Part model, mm, in its own coordinate system. Give positions to 0.01 mm unless a question says otherwise; leave off trailing zeros. Order: outer loops, then holes, each group sorted by start corner. A loop starts at its lowest first (then second) coordinate and runs counter-clockwise, first axis right, second up. Notation, with made-up numbers: M -8,39 L -4,39 A8 ccw -4,53 Z; hole C 18.25,31.5 d11. An arc over 180 degrees is marked long. Answer as a JSON object with one key per item and string values.
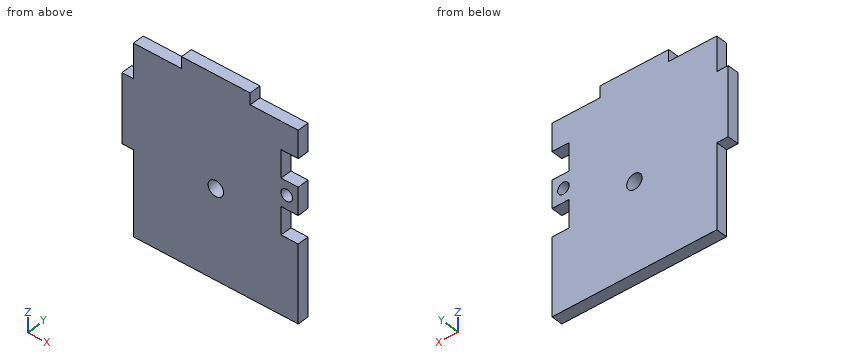
from build123d import *

# Parameters (mm, degrees)
BOSS_EXTRUDE1_DEPTH  = 3.175
M3_CLEARANCE_HOLE1_D = 3.2
SKETCH4_R            = 2.1336
CUT_EXTRUDE1_DEPTH   = 70.232936135


with BuildPart() as part:
    # Sketch1 → Boss-Extrude1 (new body)
    with BuildSketch(Plane(origin=(0, 0, 0), x_dir=(1, 0, 0), z_dir=(0, 1, 0))):
        Polygon((0, 0), (13.335, 0), (13.335, -3.175), (32.385, -3.175), (32.385, 0), (45.72, 0), (45.72, 7.62), (40.9575, 7.62), (40.9575, 15.24), (45.72, 15.24), (45.72, 22.86), (40.9575, 22.86), (40.9575, 30.48), (45.72, 30.48), (45.72, 51.8922), (0, 51.8922), (0, 28.575), (-3.175, 28.575), (-3.175, 9.525), (0, 9.525), align=None)
    extrude(amount=BOSS_EXTRUDE1_DEPTH)

    # M3 Clearance Hole1 (through all)
    with Locations(Plane(origin=(0, 3.175, 0), x_dir=(1, 0, 0), z_dir=(0, 1, 0))):
        with Locations((42.545, 19.05)):
            Hole(M3_CLEARANCE_HOLE1_D / 2)

    # Sketch4 → Cut-Extrude1 (cut, through all)
    with BuildSketch(Plane(origin=(0, 3.175, 0), x_dir=(1, 0, 0), z_dir=(0, 1, 0))):
        with Locations(Location((22.86, 27.305, 0), (0, 0, 270))):
            Circle(SKETCH4_R)
    extrude(amount=-CUT_EXTRUDE1_DEPTH, mode=Mode.SUBTRACT)


solid = part.part
1. Cut at A-A on z = -19.05. Give the cut face in (x, y) (3 decimals).
Worked answers:
{"outline": "M -3.175,0 L 40.945,0 L 40.945,3.175 L -3.175,3.175 Z; M 44.145,0 L 45.72,0 L 45.72,3.175 L 44.145,3.175 Z"}
2. Pin check, flat tips, straight feed: P1, Ø1.6, axis at y = 1.5, z = -36, coming from the -X side; P2, Ø1.6, axis at x = 3.5, y = 1.5, coming from the +Z side; P3, Ø1.6, axis at y = 1.5, z = 2, coming from the -X side (3 decimals). Stop position of each tip, or through.
Worked answers:
{"P1": "stops at x = 0", "P2": "stops at z = 0", "P3": "stops at x = 13.335"}
3. Probe line 1 along X through (y, z) = (1.15, -19.05) (3 decimals); line 2 along Z through (x, y) = (6, 1.05); line 3 along X through (y, z) = (3.05, -24) (1 decimal). List the from-to ranges inside material, lowest first.
Worked answers:
{"line 1": "x = -3.175 to 40.945, 44.145 to 45.72", "line 2": "z = -51.89 to 0", "line 3": "x = -3.2 to 41"}
4. Cut at C-C on y = 0.6. State how many separate pieces and enclosed holes the cut face has, plus the area to 3 significant figures.
Worked answers:
{"separate pieces": "1", "enclosed holes": "2", "area": "2,400 mm^2"}
5. Cut at D-D on x = 11. Give the cut face in (y, z) (3 decimals), plus the area to 3 significant figures.
Worked answers:
{"outline": "M 0,-51.892 L 3.175,-51.892 L 3.175,0 L 0,0 Z", "area": "165 mm^2"}
6. Cut at B-B on x = 22.86. Give the cut face in (y, z) (3 decimals), plus the area to 3 significant figures.
Worked answers:
{"outline": "M 0,-51.892 L 3.175,-51.892 L 3.175,-29.439 L 0,-29.439 Z; M 0,-25.171 L 3.175,-25.171 L 3.175,3.175 L 0,3.175 Z", "area": "161 mm^2"}
